```python
from build123d import *

# Parameters (mm, degrees)
F1_DEPTH = 49.53
F2_D     = 18.161
F4_D     = 3
F4_DEPTH = 7.366
F4_TIP   = 0.9012909285
F5_D     = 3
F5_DEPTH = 10.414
F5_TIP   = 0.9012909285
F6_D     = 5.334
F6_DEPTH = 7.874
F6_TIP   = 1.6024952709


# Not quite as in the source:
# - a feature of the source that left no trace in its solid (it failed there, or was rolled back) is left out


with BuildPart() as f1:
    # F0 (on Top) → F1 (new body)
    with BuildSketch(Plane.XY):
        with BuildLine():
            Line((-17.3533273419, -13.6358096689), (-17.3533273419, -17.3533273419))
            Line((-17.3533273419, -17.3533273419), (-8.3558009158, -17.3533273419))
            Line((-8.3558009158, -17.3533273419), (-8.3558009158, -13.1286343989))
            Line((-8.3558009158, -13.1286343989), (-6.7648564214, -13.1286343989))
            Line((-6.7648564214, -13.1286343989), (-6.7648564214, -17.3533273419))
            Line((-6.7648564214, -17.3533273419), (-5.8423760003, -17.3533273419))
            Line((-5.8423760003, -17.3533273419), (-5.8423760003, -13.1286343989))
            Line((-5.8423760003, -13.1286343989), (-4.2380622245, -13.1286343989))
            Line((-4.2380622245, -13.1286343989), (-4.2380622245, -17.3533273419))
            Line((-4.2380622245, -17.3533273419), (-3.3022125219, -17.3533273419))
            Line((-3.3022125219, -17.3533273419), (-3.3022125219, -13.1286343989))
            Line((-3.3022125219, -13.1286343989), (-1.7380065905, -13.1286343989))
            Line((-1.7380065905, -13.1286343989), (-1.7380065905, -17.3533273419))
            Line((-1.7380065905, -17.3533273419), (-0.7887876064, -17.3533273419))
            Line((-0.7887876064, -17.3533273419), (-0.7887876064, -13.1286343989))
            Line((-0.7887876064, -13.1286343989), (0.7887876064, -13.1286343989))
            Line((0.7887876064, -13.1286343989), (0.7887876064, -17.3533273419))
            Line((0.7887876064, -17.3533273419), (1.7380065905, -17.3533273419))
            Line((1.7380065905, -17.3533273419), (1.7380065905, -13.1286343989))
            Line((1.7380065905, -13.1286343989), (3.3022125219, -13.1286343989))
            Line((3.3022125219, -13.1286343989), (3.3022125219, -17.3533273419))
            Line((3.3022125219, -17.3533273419), (4.2380622245, -17.3533273419))
            Line((4.2380622245, -17.3533273419), (4.2380622245, -13.1286343989))
            Line((4.2380622245, -13.1286343989), (5.8423760003, -13.1286343989))
            Line((5.8423760003, -13.1286343989), (5.8423760003, -17.3533273419))
            Line((5.8423760003, -17.3533273419), (6.7648564214, -17.3533273419))
            Line((6.7648564214, -17.3533273419), (6.7648564214, -13.1286343989))
            Line((6.7648564214, -13.1286343989), (8.3558009158, -13.1286343989))
            Line((8.3558009158, -13.1286343989), (8.3558009158, -17.3533273419))
            Line((8.3558009158, -17.3533273419), (17.3533273419, -17.3533273419))
            Line((17.3533273419, -17.3533273419), (17.3533273419, -13.6358096689))
            Line((17.3533273419, -13.6358096689), (12.8737204648, -12.9246096689))
            ThreePointArc((12.8737204648, -12.9246096689), (10.7331515862, -11.9367520182), (12.9631890301, -11.1720096689))
            Line((12.9631890301, -11.1720096689), (17.3533273419, -10.4608096689))
            Line((17.3533273419, -10.4608096689), (17.3533273419, -8.3558009158))
            Line((17.3533273419, -8.3558009158), (13.1286343989, -8.3558009158))
            Line((13.1286343989, -8.3558009158), (13.1286343989, -6.7782257029))
            Line((13.1286343989, -6.7782257029), (17.3533273419, -6.7782257029))
            Line((17.3533273419, -6.7782257029), (17.3533273419, -5.8557452818))
            Line((17.3533273419, -5.8557452818), (13.1286343989, -5.8557452818))
            Line((13.1286343989, -5.8557452818), (13.1286343989, -4.224692943))
            Line((13.1286343989, -4.224692943), (17.3533273419, -4.224692943))
            Line((17.3533273419, -4.224692943), (17.3533273419, -3.3022125219))
            Line((17.3533273419, -3.3022125219), (13.1286343989, -3.3022125219))
            Line((13.1286343989, -3.3022125219), (13.1286343989, -1.6845294646))
            Line((13.1286343989, -1.6845294646), (17.3533273419, -1.6845294646))
            Line((17.3533273419, -1.6845294646), (17.3533273419, -0.7887876064))
            Line((17.3533273419, -0.7887876064), (13.1286343989, -0.7887876064))
            Line((13.1286343989, -0.7887876064), (13.1286343989, 0.7887876064))
            Line((13.1286343989, 0.7887876064), (17.3533273419, 0.7887876064))
            Line((17.3533273419, 0.7887876064), (17.3533273419, 1.6845294646))
            Line((17.3533273419, 1.6845294646), (13.1286343989, 1.6845294646))
            Line((13.1286343989, 1.6845294646), (13.1286343989, 3.3022125219))
            Line((13.1286343989, 3.3022125219), (17.3533273419, 3.3022125219))
            Line((17.3533273419, 3.3022125219), (17.3533273419, 4.224692943))
            Line((17.3533273419, 4.224692943), (13.1286343989, 4.224692943))
            Line((13.1286343989, 4.224692943), (13.1286343989, 5.8557452818))
            Line((13.1286343989, 5.8557452818), (17.3533273419, 5.8557452818))
            Line((17.3533273419, 5.8557452818), (17.3533273419, 6.7782257029))
            Line((17.3533273419, 6.7782257029), (13.1286343989, 6.7782257029))
            Line((13.1286343989, 6.7782257029), (13.1286343989, 8.3558009158))
            Line((13.1286343989, 8.3558009158), (17.3533273419, 8.3558009158))
            Line((17.3533273419, 8.3558009158), (17.3533273419, 10.414))
            Line((17.3533273419, 10.414), (12.8887263902, 11.1252))
            ThreePointArc((12.8887263902, 11.1252), (10.7559013561, 12.1292367927), (12.9912280955, 12.8778))
            Line((12.9912280955, 12.8778), (17.3533273419, 13.589))
            Line((17.3533273419, 13.589), (17.3533273419, 17.3533273419))
            Line((17.3533273419, 17.3533273419), (-17.3533273419, 17.3533273419))
            Line((-17.3533273419, 17.3533273419), (-17.3533273419, 13.589))
            Line((-17.3533273419, 13.589), (-12.9207378963, 12.8778))
            ThreePointArc((-12.9207378963, 12.8778), (-10.7315, 12.0015), (-12.9207378963, 11.1252))
            Line((-12.9207378963, 11.1252), (-17.3533273419, 10.414))
            Line((-17.3533273419, 10.414), (-17.3533273419, 8.3558009158))
            Line((-17.3533273419, 8.3558009158), (-13.1286343989, 8.3558009158))
            Line((-13.1286343989, 8.3558009158), (-13.1286343989, 6.7782257029))
            Line((-13.1286343989, 6.7782257029), (-17.3533273419, 6.7782257029))
            Line((-17.3533273419, 6.7782257029), (-17.3533273419, 5.8557452818))
            Line((-17.3533273419, 5.8557452818), (-13.1286343989, 5.8557452818))
            Line((-13.1286343989, 5.8557452818), (-13.1286343989, 4.224692943))
            Line((-13.1286343989, 4.224692943), (-17.3533273419, 4.224692943))
            Line((-17.3533273419, 4.224692943), (-17.3533273419, 3.3022125219))
            Line((-17.3533273419, 3.3022125219), (-13.1286343989, 3.3022125219))
            Line((-13.1286343989, 3.3022125219), (-13.1286343989, 1.6845294646))
            Line((-13.1286343989, 1.6845294646), (-17.3533273419, 1.6845294646))
            Line((-17.3533273419, 1.6845294646), (-17.3533273419, 0.7887876064))
            Line((-17.3533273419, 0.7887876064), (-13.1286343989, 0.7887876064))
            Line((-13.1286343989, 0.7887876064), (-13.1286343989, -0.7887876064))
            Line((-13.1286343989, -0.7887876064), (-17.3533273419, -0.7887876064))
            Line((-17.3533273419, -0.7887876064), (-17.3533273419, -1.6845294646))
            Line((-17.3533273419, -1.6845294646), (-13.1286343989, -1.6845294646))
            Line((-13.1286343989, -1.6845294646), (-13.1286343989, -3.3022125219))
            Line((-13.1286343989, -3.3022125219), (-17.3533273419, -3.3022125219))
            Line((-17.3533273419, -3.3022125219), (-17.3533273419, -4.224692943))
            Line((-17.3533273419, -4.224692943), (-13.1286343989, -4.224692943))
            Line((-13.1286343989, -4.224692943), (-13.1286343989, -5.8557452818))
            Line((-13.1286343989, -5.8557452818), (-17.3533273419, -5.8557452818))
            Line((-17.3533273419, -5.8557452818), (-17.3533273419, -6.7782257029))
            Line((-17.3533273419, -6.7782257029), (-13.1286343989, -6.7782257029))
            Line((-13.1286343989, -6.7782257029), (-13.1286343989, -8.3558009158))
            Line((-13.1286343989, -8.3558009158), (-17.3533273419, -8.3558009158))
            Line((-17.3533273419, -8.3558009158), (-17.3533273419, -10.4608096689))
            Line((-17.3533273419, -10.4608096689), (-13.0901890301, -11.2990096689))
            ThreePointArc((-13.0901890301, -11.2990096689), (-10.8601515862, -12.0637520182), (-13.0007204648, -13.0516096689))
            Line((-13.0007204648, -13.0516096689), (-17.3533273419, -13.6358096689))
        make_face()
    extrude(amount=F1_DEPTH)

    # F2 (through all)
    with Locations(Plane(origin=(0, 0, 0), x_dir=(1, 0, 0), z_dir=(0, 0, -1))):
        with Locations((0, 0)):
            Hole(F2_D / 2)

    # F4
    with Locations(Plane(origin=(0, 17.3533273419, 0), x_dir=(-1, 0, 0), z_dir=(0, 1, 0))):
        with Locations((0.033583874, 44.765), (0.033583874, 4.765)):
            Hole(F4_D / 2, depth=F4_DEPTH)
            with Locations((0, 0, -(F4_DEPTH + F4_TIP / 2))):  # 118° drill point
                Cone(0, F4_D / 2, F4_TIP, mode=Mode.SUBTRACT)

    # F5
    with Locations(Plane(origin=(0, 17.3533273419, 0), x_dir=(-1, 0, 0), z_dir=(0, 1, 0))):
        with Locations((8.033583874, 44.765), (8.033583874, 4.765), (-7.966416126, 4.765), (-7.966416126, 44.765)):
            Hole(F5_D / 2, depth=F5_DEPTH)
            with Locations((0, 0, -(F5_DEPTH + F5_TIP / 2))):  # 118° drill point
                Cone(0, F5_D / 2, F5_TIP, mode=Mode.SUBTRACT)

    # F6
    with Locations(Plane(origin=(0, 17.3533273419, 0), x_dir=(-1, 0, 0), z_dir=(0, 1, 0))):
        with Locations((0.033583874, 24.765)):
            Hole(F6_D / 2, depth=F6_DEPTH)
            with Locations((0, 0, -(F6_DEPTH + F6_TIP / 2))):  # 118° drill point
                Cone(0, F6_D / 2, F6_TIP, mode=Mode.SUBTRACT)


solid = f1.part
```
Work out the finished part from the listing and answer in its coordinate system (mm). A direction names the side the tool comes from. Coordinates: 2 decimals unless noted, no trailing zeros. Loops run counter-clockwise (first coordinate to the right, second up) from the corner with the lowest first, then second, coordinate; pieces in that order, holes last. Notation, with made-up numbers: M -5,-37.5 L 13,-37.5 A24 cw 13,-8.5 Z; hole C 9,1.25 d4. An arc over 180 degrees is marked long. Use CSV: the item, a comma, the result in double quotes. Start each with the question number.
(1) Given pin 1 Ø1.5 at (x, y) = (-12, 12) entering from +Z; pin 2 Ø0.5 at (y, z) = (-5.5, 23) entering from +X; pin 3 Ø0.8 at (x, z) = (2.5, 32) entering from -Y, each flat-ended and moving along its own axis, determine where each tip first touches the part or whether it passes through.
(2) For a pull along Z with two mould halves and no side action, classify faces 5 (the face through (17.353, 15, 24)), 6 (the face through (-8.3, 6.2, 4.8)) as +Z half, -Z half, draft (parallel to the pull), parting line (faces both ways), or undercut.
(3) Find section B-B, the plane x = -11.5. Give the vertices of the cut face in (y, z), then the cut area to 3 significant figures.
(4) For faces 1 (the face through (13.129, -8, 24)), 2 (the face through (-15, -6.778, 24)), 3 (the face through (0, 9.24, 5.02)), 4 (the face through (-4.238, -15, 24)), determine the directions among +Z, -Z, +X, -X, +Y, -Y from which every point of the face is accessible in a straight line to the end or side of a thin tool.
(5) Consider line 1 (Y direction, x = 12, z = 20); line 2 (Y direction, x = 11.5, z = 18.5); line 3 (Y direction, x = -3, z = 6). Determine where each line is inside the solid, lowest interval first.
(6) Find section A-A, the plane y = 0. Give the vertices of the cut face in (x, z).
Recorded:
1,pin 1,"passes through"
1,pin 2,"stops at x = 13.13"
1,pin 3,"stops at y = -13.13"
2,face 5,"draft"
2,face 6,"undercut"
3,outline,"M -17.35,0 L -13.23,0 L -13.23,49.53 L -17.35,49.53 Z; M -11.02,0 L 10.83,0 L 10.83,49.53 L -11.02,49.53 Z; M 13.17,0 L 17.35,0 L 17.35,49.53 L 13.17,49.53 Z"
3,area,"1,490 mm^2"
4,face 1,"+Z, -Z, +X"
4,face 2,"+Z, -Z, -X"
4,face 3,"+Y"
4,face 4,"+Z, -Z, -Y"
5,line 1,"y = -17.35 to -13.27, -10.73 to 10.79, 13.32 to 17.35"
5,line 2,"y = -17.35 to -13.17, -10.83 to 10.9, 13.21 to 17.35"
5,line 3,"y = -13.13 to -8.57, 8.57 to 17.35"
6,outline,"M -13.13,0 L -9.08,0 L -9.08,49.53 L -13.13,49.53 Z; M 9.08,0 L 13.13,0 L 13.13,49.53 L 9.08,49.53 Z"
